Source: CAD feature listing. Evaluate the final solid. Frame: model axes, mm. A direction names the side the tool comes from. Round coordinates to 2 decimals unless told otherwise and drop trailing zeros. Order: outer loops, then holes, each group sorted by start corner. A loop starts at its lowest first (then second) coordinate and runs counter-clockwise, first axis right, second up. Notation, with made-up numbers: (78.5, 73) - (101.5, 73) arc R19 ccw to (101.5, 91) - close; hole circle Ø3 at (37, 1). An arc over 180 degrees is marked (long way). Put each result on its own line as item: value. Start each with the question number.
1) Line query: probe 1 along Z at (x, y) = (-5.25, -0.75); probe 2 along Y at (x, z) = (-10.25, 50.5); probe 3 along Z at (x, y) = (-3.5, 5.5). Output: solid intervals per line, ascending. Write a range as [from, to].
2) Access query for faces 1 (the face through (-7, 0, 49)), 2 (the face through (-6.66, -3.07, 31.05)), 3 (the face through (-7, 9, 41.5)), 4 (the face through (-7, 6, 51.5)), 5 (the face through (-7, 0, 20)). Directions: +Z, -Z, +X, -X, +Y, -Y. A direction counts if a zero-diameter tool reaches every point of the face in a straight line with its end or side. Return the directions, or none.
3) Section A-A on z = 49.5. Output: boundary loops of the cut face in (x, y), then the cut area to 3 significant figures.
4) Mould query, pull axis Z, two halves, no side actions, for faces 6 (the face through (-6.66, 2.4, 14.07)), 7 (the face through (-7, 11.6, 48)), 8 (the face through (-6.66, -3.05, 42.93)). Classes: +Z half, -Z half, draft (parallel to the pull), parting line (faces both ways), or undercut.
5) Contact query for flat-ended pins moving along their axis: P1, Ø2, axis at x = -6.5, z = 30.5, coming from the +Y side; P2, Ø6, axis at x = -9.5, z = 17, coming from the -Y side; P3, Ø1, axis at x = -6.5, y = -1.5, coming from the -Z side; P4, Ø2, axis at x = -4, z = 47.5, coming from the -Y side. Output: stop coordinate, or through.
6) Section B-B on y = -1. Output: boundary loops of the cut face in (x, z).
7) Section D-D on y = 4. Output: boundary loops of the cut face in (x, z), then the cut area to 3 significant figures.
```python
from build123d import *

# Parameters (mm, degrees)
F1_DEPTH = 13.5
F2_R     = 2
F3_R     = 1.49999
F4_ANGLE = 90
F5_ANGLE = 270


# Not quite as in the source:
# - a fillet or chamfer is up to 0.001 mm smaller than in the source, because OpenCascade refuses the exact size


with BuildPart() as f1:
    # F0 (on Top) → F1 (new body)
    with BuildSketch(Plane.XY):
        Polygon((0, 12.5), (0, 0), (3, 0), (3, 38), (8.6, 38), (8.6, 28), (11.6, 28), (11.6, 41), (0, 41), (0, 32), (-2, 32), (-2, 34.5), (-3.5, 34.5), (-3.5, 29), (0, 29), (0, 15.5), (-2, 15.5), (-2, 18), (-3.5, 18), (-3.5, 12.5), align=None)
    extrude(amount=F1_DEPTH)

    # F2
    f2_edges = [f1.edges().sort_by_distance(p)[0] for p in [
        (0, 41, 6.75),
        (11.6, 41, 6.75),
        (11.6, 28, 6.75),
        (3, 0, 6.75),
    ]]
    fillet(f2_edges, radius=F2_R)

    # F3 (radius 1.5 in the source; OpenCascade refuses exactly that, so slightly less here)
    f3_edges = [f1.edges().sort_by_distance(p)[0] for p in [
        (-3.5, 34.5, 6.75),
        (-3.5, 29, 6.75),
        (-3.5, 18, 6.75),
        (-3.5, 12.5, 6.75),
    ]]
    fillet(f3_edges, radius=F3_R)


with BuildPart() as f1_1:
    # F4: moved
    add(f1.part.rotate(Axis((0, 6.25, 13.5), (0, 1, 0)), F4_ANGLE))


with BuildPart() as f1_2:
    # F5: moved
    add(f1_1.part.rotate(Axis((-6.75, 0, 13.5), (-1, 0, 0)), F5_ANGLE))


solid = f1_2.part
```
Answer sheet:
1. probe 1: [26, 29], [42.5, 45.5]
1. probe 2: [0, 3], [8.6, 11.6]
1. probe 3: [51.5, 54.5]
2. face 1: +Z, +X, -X
2. face 2: +X, -X, -Y
2. face 3: -Z, +X, -X, +Y
2. face 4: -Z, +X, -X
2. face 5: -Z, +X, -X, -Y
3. outline: (-13.5, 0) - (0, 0) - (0, 3) - (-13.5, 3) - close; (-13.5, 8.6) - (0, 8.6) - (0, 11.6) - (-13.5, 11.6) - close
3. area: 81.0 mm^2
4. face 6: -Z half
4. face 7: draft
4. face 8: undercut
5. P1: y = 3
5. P2: y = 0
5. P3: z = 26
5. P4: y = -3.5
6. outline: (-13.5, 26) - (0, 26) - (0, 29) - (-13.5, 29) - close; (-13.5, 42.5) - (0, 42.5) - (0, 45.5) - (-13.5, 45.5) - close
7. outline: (-13.5, 51.5) - (0, 51.5) - (0, 54.5) - (-13.5, 54.5) - close
7. area: 40.5 mm^2
